Check sheet for the modelled part. Datum: model origin and axes. Units: mm. A direction names the side the tool comes from. Coordinates: 2 decimals unless noted, no trailing zeros. Order: outer loops, then holes, each group sorted by start corner. A loop starts at its lowest first (then second) coordinate and runs counter-clockwise, first axis right, second up.
1. Cross-section at C-C (x = -71). Enter the section's corners in (y, z).
2. Gauge pin test, flat ends, axial feed: pin 1 Ø2 at (x, y) = (-62.5, 12.5) entering from -Z; pin 2 Ø2.5 at (y, z) = (16.5, 0.5) entering from +X; pin 3 Ø11.5 at (x, y) = (78.5, 11.5) entering from -Z; pin 4 Ø15 at (x, y) = (-46.5, 3) entering from +Z. Record the tip position at first contact, or that the pin passes through.
3. Cross-section at B-B (z = 26). Enter the section's corners in (x, y) (3 decimals), then the cut area to 4 significant figures.
4. Set-up check for faces 4 (the cylindrical face through (-69.345, 15.068, 5.528)), 5 (the flat face through (70.75, 10, 22)), 6 (the flat face through (-63, 17, 1.1)), 7 (the cylindrical face through (68.71, 12.47, 0.11)), 8 (the flat face through (72.825, 10, 22)): record each of +Z, -Z, +X, -X, +Y, -Y from which the full face is reachable in a straight line by a thin tool's end or side.
5. Thickness scan on line 1 (X direction, y = 15, z = 26) (3 decimals); line 2 (Y direction, x = -50.5, z = 2); line 3 (Y direction, x = -77.5, z = 6.15). Record the ranges inside material, lowest first.
6. Cross-section at A-A (x = -50.5). Enter the section's corners in (y, z).
7. Draft check along Y on faces 1 (the flat face through (79, 10, 11)), 2 (the flat face through (6, 25, 2)), 3 (the flat face through (29, 23.25, 0)). Enter one of: released by +Y, released by -Y, zero draft, split by the parting line, or undercut.
```python
from build123d import *

# Parameters (mm, degrees)
SKETCH1_W           = 175
SKETCH1_H           = 15
BOSS_EXTRUDE1_DEPTH = 25
CUT_EXTRUDE1_REACH  = 17
SKETCH3_R           = 4.6
SKETCH3_R_2         = 8.05
SKETCH3_R_3         = 1.3
SKETCH3_3_R         = 8.55
SKETCH3_3_R_2       = 4.6
CUT_EXTRUDE2_DEPTH  = 4
CUT_EXTRUDE3_DEPTH  = 1.1
CUT_EXTRUDE4_REACH  = 27
SKETCH5_R           = 1.3
CUT_EXTRUDE6_REACH  = 17
SKETCH8_W           = 175
SKETCH8_H           = 15
BOSS_EXTRUDE2_DEPTH = 5
SKETCH9_W           = 16.75
SKETCH9_H           = 30
BOSS_EXTRUDE3_DEPTH = 30
SKETCH10_R          = 1.1
CUT_EXTRUDE7_DEPTH  = 30
FILLET1_R           = 10


with BuildPart() as part:
    # Sketch1 → Boss-Extrude1 (new body)
    with BuildSketch(Plane(origin=(0, 0, 0), x_dir=(1, 0, 0), z_dir=(0, 1, 0))):
        Rectangle(SKETCH1_W, SKETCH1_H)
    extrude(amount=BOSS_EXTRUDE1_DEPTH)

    # Sketch3 → Cut-Extrude1 (cut, up to next)
    with BuildSketch(Plane.XY.offset(7.5), mode=Mode.PRIVATE) as cut_extrude1_sk1:
        with Locations((-77.5, 12.5)):
            Circle(SKETCH3_R)
    cut_extrude1_tool1 = extrude(cut_extrude1_sk1.sketch, amount=-CUT_EXTRUDE1_REACH, mode=Mode.PRIVATE) & part.part
    add(cut_extrude1_tool1.solids().sort_by_distance((-77.5, 12.5, 7.5))[0], mode=Mode.SUBTRACT)
    # Sketch3 → Cut-Extrude1 (cut, up to next)
    with BuildSketch(Plane.XY.offset(7.5), mode=Mode.PRIVATE) as cut_extrude1_sk2:
        with Locations((-50.5, 12.5)):
            Circle(SKETCH3_R_2)
    cut_extrude1_tool2 = extrude(cut_extrude1_sk2.sketch, amount=-CUT_EXTRUDE1_REACH, mode=Mode.PRIVATE) & part.part
    add(cut_extrude1_tool2.solids().sort_by_distance((-50.5, 12.5, 7.5))[0], mode=Mode.SUBTRACT)
    # Sketch3 → Cut-Extrude1 (cut, up to next)
    with BuildSketch(Plane.XY.offset(7.5), mode=Mode.PRIVATE) as cut_extrude1_sk3:
        with Locations((-24.5, 12.5)):
            Circle(SKETCH3_R_2)
    cut_extrude1_tool3 = extrude(cut_extrude1_sk3.sketch, amount=-CUT_EXTRUDE1_REACH, mode=Mode.PRIVATE) & part.part
    add(cut_extrude1_tool3.solids().sort_by_distance((-24.5, 12.5, 7.5))[0], mode=Mode.SUBTRACT)
    # Sketch3 → Cut-Extrude1 (cut, up to next)
    with BuildSketch(Plane.XY.offset(7.5), mode=Mode.PRIVATE) as cut_extrude1_sk4:
        with Locations((-62.5, 12.5)):
            Circle(SKETCH3_R_3)
    cut_extrude1_tool4 = extrude(cut_extrude1_sk4.sketch, amount=-CUT_EXTRUDE1_REACH, mode=Mode.PRIVATE) & part.part
    add(cut_extrude1_tool4.solids().sort_by_distance((-62.5, 12.5, 7.5))[0], mode=Mode.SUBTRACT)

    # Sketch3<3> → Cut-Extrude2 (cut)
    with BuildSketch(Plane.XY.offset(7.5)):
        with Locations((-77.5, 12.5)):
            Circle(SKETCH3_3_R)
        with Locations((-77.5, 12.5)):
            Circle(SKETCH3_3_R_2, mode=Mode.SUBTRACT)
    extrude(amount=-CUT_EXTRUDE2_DEPTH, mode=Mode.SUBTRACT)

    # Sketch4 → Cut-Extrude3 (cut, symmetric)
    with BuildSketch(Plane.XY):
        Polygon((-59.9, 10.9988893), (-59.9, 14.0011107), (-62.5, 15.5022214), (-65.1, 14.0011107), (-65.1, 10.9988893), (-62.5, 9.4977786), align=None)
        Polygon((-59.9, 25), (-59.9, 14.0011107), (-62.5, 15.5022214), (-65.1, 14.0011107), (-65.1, 25), align=None)
    extrude(amount=CUT_EXTRUDE3_DEPTH, both=True, mode=Mode.SUBTRACT)

    # Sketch5 → Cut-Extrude4 (cut, up to next)
    with BuildSketch(Plane(origin=(0, 25, 0), x_dir=(1, 0, 0), z_dir=(0, 1, 0)), mode=Mode.PRIVATE) as cut_extrude4_sk1:
        Circle(SKETCH5_R)
    cut_extrude4_tool1 = extrude(cut_extrude4_sk1.sketch, amount=-CUT_EXTRUDE4_REACH, mode=Mode.PRIVATE) & part.part
    add(cut_extrude4_tool1.solids().sort_by_distance((0, 25, 0))[0], mode=Mode.SUBTRACT)

    # Sketch6 → Cut-Extrude6 (cut, up to next)
    with BuildSketch(Plane.XY.offset(7.5), mode=Mode.PRIVATE) as cut_extrude6_sk1:
        with BuildLine():
            Line((57, 23), (0, 23))
            ThreePointArc((0, 23), (-11.5, 11.5), (0, 0))
            Line((0, 0), (57, 0))
            ThreePointArc((57, 0), (68.5, 11.5), (57, 23))
        make_face()
    cut_extrude6_tool1 = extrude(cut_extrude6_sk1.sketch, amount=-CUT_EXTRUDE6_REACH, mode=Mode.PRIVATE) & part.part
    add(cut_extrude6_tool1.solids().sort_by_distance((28.5, 11.5, 7.5))[0], mode=Mode.SUBTRACT)
    # Sketch6 → Cut-Extrude6 (cut, up to next)
    with BuildSketch(Plane.XY.offset(7.5), mode=Mode.PRIVATE) as cut_extrude6_sk2:
        with BuildLine():
            ThreePointArc((0, 0), (-11.5, 11.5), (0, 23))
            Line((0, 23), (57, 23))
            ThreePointArc((57, 23), (68.5, 11.5), (57, 0))
            Line((57, 0), (59.41091269, 0))
            ThreePointArc((59.41091269, 0), (68.687332887, 12.711919964), (57, 23.25))
            Line((57, 23.25), (0, 23.25))
            ThreePointArc((0, 23.25), (-11.687332887, 12.711919964), (-2.41091269, 0))
            Line((-2.41091269, 0), (0, 0))
        make_face()
    cut_extrude6_tool2 = extrude(cut_extrude6_sk2.sketch, amount=-CUT_EXTRUDE6_REACH, mode=Mode.PRIVATE) & part.part
    add(cut_extrude6_tool2.solids().sort_by_distance((68.603989, 12.703278, 7.5))[0], mode=Mode.SUBTRACT)

    # Sketch8 → Boss-Extrude2 (add)
    with BuildSketch(Plane.XZ):
        Rectangle(SKETCH8_W, SKETCH8_H)
    extrude(amount=BOSS_EXTRUDE2_DEPTH)

    # Sketch9 → Boss-Extrude3 (add)
    with BuildSketch(Plane.XY.offset(7.5)):
        with Locations((79.125, 10)):
            Rectangle(SKETCH9_W, SKETCH9_H)
    extrude(amount=BOSS_EXTRUDE3_DEPTH)

    # Sketch10 → Cut-Extrude7 (cut)
    with BuildSketch(Plane(origin=(0, 25, 0), x_dir=(1, 0, 0), z_dir=(0, 1, 0))):
        with Locations((79.125, -8.45)):
            Circle(SKETCH10_R)
        with BuildLine():
            Line((73.825, -34), (84.425, -34))
            ThreePointArc((84.425, -34), (85.132106781, -33.707106781), (85.425, -33))
            Line((85.425, -33), (85.425, -12))
            ThreePointArc((85.425, -12), (85.132106781, -11.292893219), (84.425, -11))
            Line((84.425, -11), (73.825, -11))
            ThreePointArc((73.825, -11), (73.117893219, -11.292893219), (72.825, -12))
            Line((72.825, -12), (72.825, -33))
            ThreePointArc((72.825, -33), (73.117893219, -33.707106781), (73.825, -34))
        make_face()
    extrude(amount=-CUT_EXTRUDE7_DEPTH, mode=Mode.SUBTRACT)

    # Fillet1
    fillet1_edges = [part.edges().sort_by_distance(p)[0] for p in [
        (87.5, 10, -7.5),
    ]]
    fillet(fillet1_edges, radius=FILLET1_R)


solid = part.part
```
Data:
1. outline: (-5, -7.5) - (25, -7.5) - (25, 7.5) - (18.05, 7.5) - (18.05, 3.5) - (6.95, 3.5) - (6.95, 7.5) - (-5, 7.5) - close
2. pin 1: passes through
2. pin 2: stops at x = 87.47
2. pin 3: stops at z = -7.5
2. pin 4: stops at z = 7.5
3. outline: (70.75, -5) - (72.825, -5) - (72.825, 25) - (70.75, 25) - close; (85.425, -5) - (87.5, -5) - (87.5, 25) - (85.425, 25) - close
3. area: 124.5 mm2
4. face 4: +Z
4. face 5: +Z, -X, +Y, -Y
4. face 6: +Y
4. face 7: +Z, -Z
4. face 8: +Y, -Y
5. line 1: x = 70.75 to 72.825, 85.425 to 87.5
5. line 2: y = -5 to 4.45, 20.55 to 25
5. line 3: y = -5 to 3.95, 21.05 to 25
6. outline: (-5, -7.5) - (4.45, -7.5) - (4.45, 7.5) - (-5, 7.5) - close; (20.55, -7.5) - (25, -7.5) - (25, 7.5) - (20.55, 7.5) - close
7. face 1: zero draft
7. face 2: released by +Y
7. face 3: undercut
